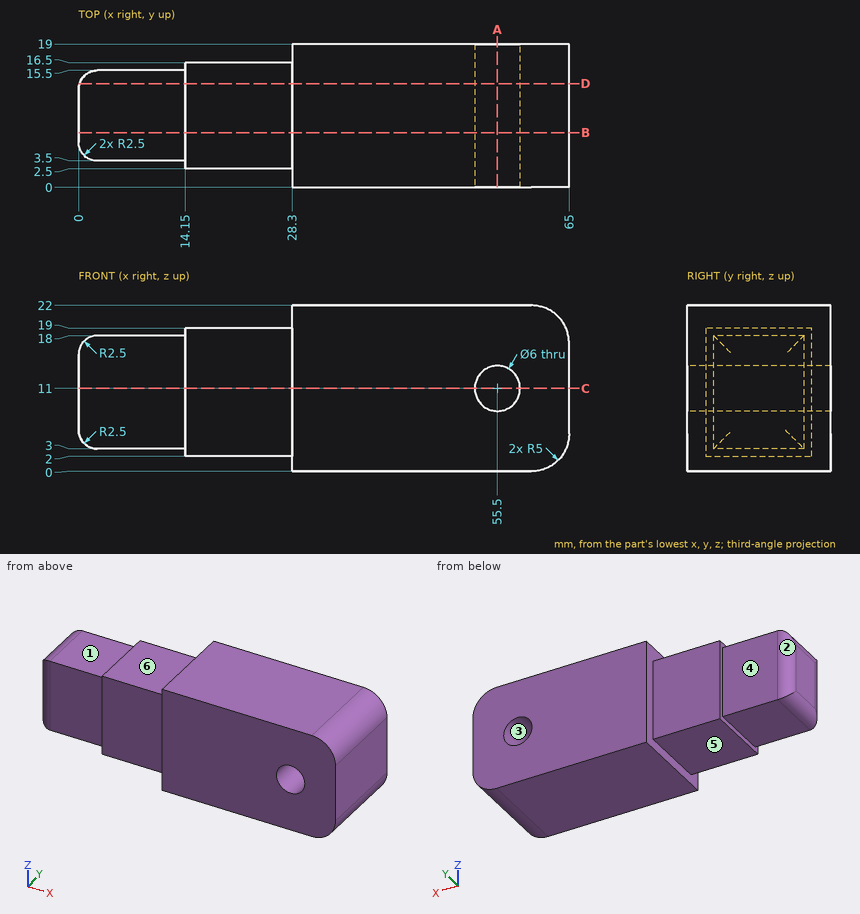
Geometry check sheet. Reference: drawing and pictorial views, mm from the part's lowest x, y, z. A direction names the side the tool comes from. Coordinates: 2 decimals unless noted, no trailing zeros. Write each loop counter-clockwise with the first axis right and the second up, starting at its lowest first coordinate (ties: lowest second). Pieces come first, ordered by that corner, then holes.
Item 1: Cross-section at D-D on y = 13.75. Record the boundary of the cut face in (x, z), then the cut area to 3 significant figures.
Numbers:
outline: (0.12, 4.75) arc R2.5 ccw to (2.5, 3) - (14.15, 3) - (14.15, 2) - (28.3, 2) - (28.3, 0) - (60, 0) arc R5 ccw to (65, 5) - (65, 17) arc R5 ccw to (60, 22) - (28.3, 22) - (28.3, 19) - (14.15, 19) - (14.15, 18) - (2.5, 18) arc R2.5 ccw to (0.12, 16.25) - close; hole circle Ø6 at (55.5, 11)
area: 1,220 mm2
Item 2: Cross-section at A-A on x = 55.5. Record the boundary of the cut face in (y, z).
Numbers:
outline: (0, 0) - (19, 0) - (19, 8) - (0, 8) - close; (0, 14) - (19, 14) - (19, 22) - (0, 22) - close
Item 3: Cross-section at B-B on y = 7.25. Record the boundary of the cut face in (x, z), then the cut area to 3 significant figures.
Numbers:
outline: (0, 5.5) arc R2.5 ccw to (2.5, 3) - (14.15, 3) - (14.15, 2) - (28.3, 2) - (28.3, 0) - (60, 0) arc R5 ccw to (65, 5) - (65, 17) arc R5 ccw to (60, 22) - (28.3, 22) - (28.3, 19) - (14.15, 19) - (14.15, 18) - (2.5, 18) arc R2.5 ccw to (0, 15.5) - close; hole circle Ø6 at (55.5, 11)
area: 1,220 mm2
Item 4: Scan lines: probe 1 along Z at (x, y) = (55.5, 9.5); probe 2 along Z at (x, y) = (20.5, 14.25); probe 3 along Z at (x, y) = (56.5, 15.5). Record each from-to range of solid material in increasing order.
Numbers:
probe 1: z = 0 to 8, 14 to 22
probe 2: z = 2 to 19
probe 3: z = 0 to 8.17, 13.83 to 22
Item 5: Access from +Z, -Z, +X, -X, +Y, -Y to the whole of each face (thin tool, end or side, straight path). Record for the marked faces 4, 5 and 6.
Numbers:
face 4: +Z, -Z, -X, +Y
face 5: -Z, -X, +Y, -Y
face 6: +Z, -X, +Y, -Y
Item 6: Cross-section at C-C on z = 11. Record the boundary of the cut face in (x, y).
Numbers:
outline: (0, 6) arc R2.5 ccw to (2.5, 3.5) - (14.15, 3.5) - (14.15, 2.5) - (28.3, 2.5) - (28.3, 0) - (52.5, 0) - (52.5, 19) - (28.3, 19) - (28.3, 16.5) - (14.15, 16.5) - (14.15, 15.5) - (2.5, 15.5) arc R2.5 ccw to (0, 13) - close; (58.5, 0) - (65, 0) - (65, 19) - (58.5, 19) - close
Item 7: Mould release check, pull along X, two halves, no side actions. Record for the marked faces 1, 2 and 3: released by +X, released by -X, zero draft, split by the parting line, or undercut.
Numbers:
face 1: zero draft
face 2: released by -X
face 3: undercut
Item 8: Depth check by flat-ended pin: pin 1 Ø10 at (y, z) = (6, 2.5) entering from +X; pin 2 Ø13 at (x, z) = (6.5, 13.5) entering from -Y; pin 3 Ø11 at (x, y) = (22.5, 6.5) entering from +Z; pin 4 Ø3.5 at (x, y) = (9, 7.5) entering from +Z. Enter the tip coordinate at first touch or a pass-through.
Numbers:
pin 1: stops at x = 65
pin 2: stops at y = 3.5
pin 3: stops at z = 19
pin 4: stops at z = 18
